Design review of the part built by this model. Coordinates are the model's own, in mm. A direction names the side the tool comes from. Give positions to 0.01 mm unless a question says otherwise; leave off trailing zeros. Write each loop counter-clockwise with the first axis right and the second up, starting at its lowest first coordinate (ties: lowest second). Pieces come first, ordered by that corner, then holes. Notation, with made-up numbers: (79.5, 29) -> (92.5, 29) arc R17 ccw to (92.5, 43) -> close; hole circle Ø7 at (61.5, 21.5). An arc over 180 degrees is marked (long way). Return JSON: item names as keys, results as strings. Group by question number.
from build123d import *

# Parameters (mm, degrees)
BOSS_EXTRUDE1_DEPTH = 25.4


with BuildPart() as part:
    # Sketch1 → Boss-Extrude1 (new body)
    with BuildSketch(Plane(origin=(0, 0, 0), x_dir=(1, 0, 0), z_dir=(0, 1, 0))):
        Polygon((-123.169565917, -23.329882989), (126.830434083, -23.329882989), (108.874840712, 7.770117011), (-105.213972545, 7.770117011), align=None)
        Polygon((155.808230769, 26.861133162), (126.830434083, -23.329882989), (108.874840712, 7.770117011), (128.874840712, 42.411133162), align=None)
    extrude(amount=BOSS_EXTRUDE1_DEPTH)


solid = part.part
Q1. For L1, parallel to Z at x = -74, y = 23.5; L2, parallel to X at y = 11, z = -35; L3, parallel to X at y = 2.5, z = 20.5, list the stretches that pass through material, from the lowest coordinate up. Write a range as from..to.
Q2. Tool access review of faces 1 (the face through (14, 25.4, 5)), 2 (the face through (3, 13, -7.77)): name each direction out of +Z, -Z, +X, -X, +Y, -Y from which nothing blocks a thin tool from reaching the whole face with its end or side.
Q3. Take a section at C-C, the plane z = -17. Give the boundary of the cut face in (x, y).
Q4. Insertion check: pin 1 (1.5 mm diameter, centred on y = 19, z = 7, fed in from +X); pin 2 (8 mm diameter, centred on y = 14, z = -14.5, fed in from +X); pin 3 (12.5 mm diameter, centred on x = 14, y = 18, fed in from -Z). Each pin has a flat end and moves straight along its axis. Give the tip position at first contact, or say it passes through.
Q5. Take a section at B-B, the plane x = -14.5. Give the boundary of the cut face in (y, z), plus the area to 3 significant figures.
Q6. Take a section at A-A, the plane y = 7.75. Give the boundary of the cut face in (x, z).
Final values:
{
 "1": {"L1": "z = -7.77..23.33", "L2": "x = 124.6..141.71", "L3": "x = -121.54..128.46"},
 "2": {"face 1": "+Z, -Z, +X, -X, +Y", "face 2": "-Z, -X, +Y, -Y"},
 "3": {"outline": "(114.2, 0) -> (150.11, 0) -> (150.11, 25.4) -> (114.2, 25.4) -> close"},
 "4": {"pin 1": "stops at x = 136.69", "pin 2": "stops at x = 150.98", "pin 3": "stops at z = -7.77"},
 "5": {"outline": "(0, -7.77) -> (25.4, -7.77) -> (25.4, 23.33) -> (0, 23.33) -> close", "area": "790 mm²"},
 "6": {"outline": "(-123.17, 23.33) -> (-105.21, -7.77) -> (108.87, -7.77) -> (128.87, -42.41) -> (155.81, -26.86) -> (126.83, 23.33) -> close"}
}
